Source: CAD feature listing. Evaluate the final solid. Frame: model axes, mm. A direction names the side the tool comes from. Round coordinates to 2 decimals unless told otherwise and drop trailing zeros. Order: outer loops, then holes, each group sorted by start corner. A loop starts at its lowest first (then second) coordinate and runs counter-clockwise, first axis right, second up. Notation, with made-up numbers: (-31, 52.5) - (-12, 52.5) arc R25 ccw to (-12, 71.5) - close; hole circle Ø8 at (62, 79). An arc over 180 degrees is marked (long way). Return JSON: item names as keys, results as strings. Group by question number.
1) Access query for faces 4 (the flat face through (0, -2, 8)), 5 (the cylindrical face through (0, -11.6, 2)), 6 (the flat face through (-7.24, -7.11, 1.97)). Directions: +Z, -Z, +X, -X, +Y, -Y. A direction counts if a zero-diameter tool reaches every point of the face in a straight line with its end or side. Return the directions, or none.
2) Contact query for flat-ended pins moving along their axis: P1, Ø2, axis at y = -9, z = 1, coming from the +X side; P2, Ø2, axis at y = -9.5, z = 1.5, coming from the -X side. Output: stop coordinate, or through.
3) Section A-A, the plane x = 0. Return loops of the section in (y, z), plus the area to 3 significant figures.
4) Mould query, pull axis X, two halves, no side actions, for faces 1 (the cylindrical face through (0, -6.4, 2)), 2 (the flat face through (10, 0, 6)), 3 (the flat face through (0, -6, 4)). Classes: pulls with the +X half, pulls with the -X half, needs draft (parallel to the pull), parting line crosses it, or undercut.
5) Section C-C, the plane z = 8.75. Return loops of the section in (x, y).
6) Section B-B, the plane z = 2.5. Return loops of the section in (x, y), plus the area to 3 significant figures.
7) Ray query, line 1 (Z direction, x = -6, y = -2.25); line 2 (Y direction, x = 5.5, z = 4.25); line 3 (X direction, y = -9.75, z = 1.75). Return the intervals inside material, ascending. Write a range as from..to.
8) Section D-D, the plane x = -2.5. Return loops of the section in (y, z).
```python
from build123d import *

# Parameters (mm, degrees)
F1_DEPTH = 4
F0_W     = 20
F0_H     = 4
F2_DEPTH = 13


with BuildPart() as f1:
    # F0 (on Top) → F1 (new body)
    with BuildSketch(Plane.XY):
        with BuildLine():
            Line((4.399958, -12.374947), (10, -2))
            Line((10, -2), (-10, -2))
            Line((-10, -2), (-4.399958, -12.374947))
            ThreePointArc((-4.399958, -12.374947), (0, -15), (4.399958, -12.374947))
        make_face()
        with BuildLine():
            Line((-1.6, -10), (-1.6, -8))
            ThreePointArc((-1.6, -8), (0, -6.4), (1.6, -8))
            Line((1.6, -8), (1.6, -10))
            ThreePointArc((1.6, -10), (0, -11.6), (-1.6, -10))
        make_face(mode=Mode.SUBTRACT)
    extrude(amount=F1_DEPTH)

    # F0 (on Top) → F2 (join)
    with BuildSketch(Plane.XY):
        Rectangle(F0_W, F0_H)
    extrude(amount=F2_DEPTH)


solid = f1.part
```
Geometry check:
{
 "1": {"face 4": "+Z, +X, -X, -Y", "face 5": "+Z, -Z", "face 6": "+Z, -Z, -X, -Y"},
 "2": {"P1": "x = 6.76", "P2": "x = -6.49"},
 "3": {"outline": "(-15, 0) - (-11.6, 0) - (-11.6, 4) - (-15, 4) - close; (-6.4, 0) - (2, 0) - (2, 13) - (-2, 13) - (-2, 4) - (-6.4, 4) - close", "area": "83.2 mm2"},
 "4": {"face 1": "undercut", "face 2": "pulls with the +X half", "face 3": "needs draft"},
 "5": {"outline": "(-10, -2) - (10, -2) - (10, 2) - (-10, 2) - close"},
 "6": {"outline": "(-10, -2) - (-4.4, -12.37) arc R5 ccw to (4.4, -12.37) - (10, -2) - (10, 2) - (-10, 2) - close; hole (-1.6, -10) arc R1.6 ccw to (1.6, -10) - (1.6, -8) arc R1.6 ccw to (-1.6, -8) - close", "area": "231 mm2"},
 "7": {"line 1": "0..4", "line 2": "-2..2", "line 3": "-5.82..-1.6, 1.6..5.82"},
 "8": {"outline": "(-14.33, 0) - (2, 0) - (2, 13) - (-2, 13) - (-2, 4) - (-14.33, 4) - close"}
}
